Check sheet for the modelled part. Datum: model origin and axes. Units: mm. A direction names the side the tool comes from. Round coordinates to 2 decimals unless told otherwise and drop trailing zeros. Loops run counter-clockwise (first coordinate to the right, second up) from the corner with the lowest first, then second, coordinate; pieces in that order, holes last. Notation, with made-up numbers: (-24, 4) - (-2, 4) arc R12 ccw to (-2, 16) - close; hole circle Ø3 at (-14, 48.5). An arc over 180 degrees is marked (long way). Return JSON: item names as keys, results as strings.
from build123d import *

# Parameters (mm, degrees)
SKETCH_1_R          = 26
EXTRUDE_1_DEPTH     = 10
SKETCH_3_R          = 29
CUT_EXTRUDE_1_DEPTH = 6
SKETCH_4_W          = 40
SKETCH_4_H          = 12
EXTRUDE_2_DEPTH     = 12
SKETCH_5_W          = 40
SKETCH_5_H          = 12
EXTRUDE_3_DEPTH     = 2
SKETCH_6_W          = 40
SKETCH_6_H          = 12
EXTRUDE_4_DEPTH     = 3
CHAMFER_1_SIZE      = 14
SKETCH_7_R          = 1.7
CUT_EXTRUDE_2_DEPTH = 14
SKETCH_8_R          = 2.15
SKETCH_8_R_2        = 2.165
CUT_EXTRUDE_3_DEPTH = 6
SKETCH_9_W          = 40
SKETCH_9_H          = 12
CUT_EXTRUDE_4_DEPTH = 5
CHAMFER_2_SIZE      = 4
CHAMFER_3_SIZE      = 4
FILLET_5_R          = 10
FILLET_6_R          = 4
FILLET_7_R          = 3


with BuildPart() as part:
    # Sketch 1 → Extrude 1 (new body)
    with BuildSketch(Plane.XY):
        with BuildLine():
            Line((20, -27.158003748), (-20, -27.158003748))
            Line((-20, -27.158003748), (-20, 0.909194251))
            ThreePointArc((-20, 0.909194251), (0, 60.158003748), (20, 0.909194251))
            Line((20, 0.909194251), (20, -27.158003748))
        make_face()
        with Locations((0, 27.158003748)):
            Circle(SKETCH_1_R, mode=Mode.SUBTRACT)
    extrude(amount=EXTRUDE_1_DEPTH)

    # Sketch 3 → Cut-Extrude 1 (cut)
    with BuildSketch(Plane.XY.offset(10)):
        with Locations((0, 27.158003748)):
            Circle(SKETCH_3_R)
    extrude(amount=-CUT_EXTRUDE_1_DEPTH, mode=Mode.SUBTRACT)



with BuildPart() as body_2:
    # Sketch 4 → Extrude 2 (new body)
    with BuildSketch(Plane.XY.offset(10)):
        with Locations((0, -33.158003748)):
            Rectangle(SKETCH_4_W, SKETCH_4_H)
    extrude(amount=EXTRUDE_2_DEPTH)


with BuildPart() as part_1:
    add(part.part)

    add(body_2.part)  # Extrude 3 merges body 2
    # Sketch 5 → Extrude 3 (add)
    with BuildSketch(Plane(origin=(0, 0, 10), x_dir=(-1, 0, 0), z_dir=(0, 0, -1))):
        with Locations((0, -33.158003748)):
            Rectangle(SKETCH_5_W, SKETCH_5_H)
    extrude(amount=EXTRUDE_3_DEPTH)

    # Sketch 6 → Extrude 4 (add)
    with BuildSketch(Plane(origin=(0, -27.158003748, 0), x_dir=(1, 0, 0), z_dir=(0, 1, 0))):
        with Locations((0, -16)):
            Rectangle(SKETCH_6_W, SKETCH_6_H)
    extrude(amount=EXTRUDE_4_DEPTH)

    # Chamfer 1
    # the kernel refuses this chamfer: 14 mm, written as the material it adds along each edge
    with BuildSketch(Plane(origin=(-20, -24.158003748, 10), x_dir=(0, -0.027495876610586365, 0.9996219169112968), z_dir=(1, 0, 0))) as chamfer_1_piece_1_section:
        Polygon((CHAMFER_1_SIZE * 0.999621916911, -CHAMFER_1_SIZE * 0.0274958766106), (-CHAMFER_1_SIZE * 0.0274958766106, -CHAMFER_1_SIZE * 0.999621916911), (0, 0), align=None)
    chamfer_1_piece_1 = extrude(amount=40, mode=Mode.PRIVATE)
    chamfer_1_piece_1 = split(chamfer_1_piece_1, bisect_by=Plane(origin=(0, -19.403075602, 22), z_dir=(0, 0, -1)), keep=Keep.TOP, mode=Mode.PRIVATE)
    add(chamfer_1_piece_1)

    # Sketch 7 → Cut-Extrude 2 (cut)
    with BuildSketch(Plane(origin=(0, 0, 8), x_dir=(-1, 0, 0), z_dir=(0, 0, -1))):
        with Locations((-12, -33.833568363)):
            Circle(SKETCH_7_R)
        with Locations((12.012999622, -33.833568363)):
            Circle(SKETCH_7_R)
    extrude(amount=-CUT_EXTRUDE_2_DEPTH, mode=Mode.SUBTRACT)

    # Sketch 8 → Cut-Extrude 3 (cut)
    with BuildSketch(Plane.XY.offset(22)):
        with Locations((-12.012999622, -33.833568363)):
            Circle(SKETCH_8_R)
        with Locations((12, -33.833568363)):
            Circle(SKETCH_8_R_2)
    extrude(amount=-CUT_EXTRUDE_3_DEPTH, mode=Mode.SUBTRACT)

    # Sketch 9 → Cut-Extrude 4 (cut)
    with BuildSketch(Plane(origin=(0, 0, 8), x_dir=(-1, 0, 0), z_dir=(0, 0, -1))):
        with Locations((0, -33.158003748)):
            Rectangle(SKETCH_9_W, SKETCH_9_H)
    extrude(amount=-CUT_EXTRUDE_4_DEPTH, mode=Mode.SUBTRACT)

    # Chamfer 2
    # the kernel refuses this chamfer: 4 mm, written as the material it takes off along each edge
    with BuildSketch(Plane(origin=(30.286731952, -39.158003748, 22), x_dir=(0, 0.9996219169112968, 0.02749587661058651), z_dir=(-1, 0, 0))) as chamfer_2_piece_1:
        Polygon((CHAMFER_2_SIZE * 0.999621916911, CHAMFER_2_SIZE * 0.0274958766106), (-CHAMFER_2_SIZE * 0.0274958766106, CHAMFER_2_SIZE * 0.999621916911), (0, 0), align=None)
    extrude(amount=60.573463904, mode=Mode.SUBTRACT)

    # Chamfer 3
    chamfer_3_edges = [part_1.edges().sort_by_distance(p)[0] for p in [
        (0, -27.158003748, 0),
    ]]
    chamfer(chamfer_3_edges, length=CHAMFER_3_SIZE)

    # Fillet 5
    fillet_5_edges = [part_1.edges().sort_by_distance(p)[0] for p in [
        (-20, 0.909194251, 5),
        (20, 0.909194251, 5),
    ]]
    fillet(fillet_5_edges, radius=FILLET_5_R)

    # Fillet 6
    fillet_6_edges = [part_1.edges().sort_by_distance(p)[0] for p in [
        (0, 60.158003748, 0),
        (-20, -13.402921801, 0),
        (-20.786763819, 0.240126076, 0),
        (20.786763819, 0.240126076, 0),
        (20, -13.402921801, 0),
    ]]
    fillet(fillet_6_edges, radius=FILLET_6_R)

    # Fillet 7
    fillet_7_edges = [part_1.edges().sort_by_distance(p)[0] for p in [
        (0, -22.158003748, 22),
    ]]
    fillet(fillet_7_edges, radius=FILLET_7_R)


solid = part_1.part
Q1. Sectioned sample at B-B (y = -6). Enter the section's corners in (x, z).
Answer key:
{"outline": "(-20, 4) arc R4 ccw to (-16, 0) - (16, 0) arc R4 ccw to (20, 4) - (20, 10) - (-20, 10) - close"}
Q2. Sectioned sample at C-C (z = 8.75). Enter the section's corners in (x, y).
Answer key:
{"outline": "(-23.02, 3.52) arc R10 cw to (-20, -3.65) - (-20, -27.16) - (20, -27.16) - (20, -3.65) arc R10 cw to (23.02, 3.52) arc R33 ccw (long way) to start; hole circle Ø58 at (0, 27.16)"}
Q3. Tool access check on faces 4 (the face through (-10, -1, 10)), 5 (the face through (-11, 51, 4)), 6 (the face through (-18.797, -15.238, 1.141)). Record the directions out of +Z, -Z, +X, -X, +Y, -Y that give a thin tool (end or side, any length) a straight path to the whole face; none if there is none.
Answer key:
{"face 4": "+Z, +X, -X, +Y", "face 5": "+Z", "face 6": "-Z, -X, -Y"}
Q4. Scan lines: probe 1 along Z at (x, y) = (-9.5, 0); probe 2 along X at (y, z) = (1.5, 6.5); probe 3 along Y at (x, z) = (-4, 9.25). Record each from-to range of solid material in increasing order. Write a range as [from, to].
Answer key:
{"probe 1": "z = [0, 4]", "probe 2": "x = [-21.43, -13.52], [13.52, 21.43]", "probe 3": "y = [-27.16, -1.56], [55.88, 59.91]"}
Q5. Depth check by flat-ended pin: P1, Ø5, axis at y = 34, z = 3.5, coming from the -X side; P2, Ø10, axis at x = 9.5, z = 7.5, coming from the -Y side; P3, Ø2, axis at x = 6, y = -2, coming from the +Z side; P4, Ø12, axis at y = 28.5, z = 16.5, coming from the +X side. Enter the tip coordinate at first touch or a pass-through.
Answer key:
{"P1": "stops at x = -32.71", "P2": "stops at y = -27.16", "P3": "stops at z = 10", "P4": "passes through"}
Q6. Draft check along X on faces 1 (the face through (20, -22, 13)), 2 (the face through (-14, -34, 16)), 3 (the face through (0, -29, 22)). Enter one of: released by +X, released by -X, zero draft, split by the parting line, or undercut.
Answer key:
{"face 1": "released by +X", "face 2": "undercut", "face 3": "zero draft"}
Q7. Sectioned sample at A-A (x = 0). Enter the section's corners in (y, z).
Answer key:
{"outline": "(-39.16, 13) - (-27.16, 13) - (-27.16, 4) - (-23.16, 0) - (1.16, 0) - (1.16, 4) - (-1.84, 4) - (-1.84, 10) - (-10.16, 10) - (-21.28, 21.12) arc R3 ccw to (-23.4, 22) - (-35.16, 22) - (-39.16, 18) - close; (53.16, 0) - (56.16, 0) arc R4 ccw to (60.16, 4) - (60.16, 10) - (56.16, 10) - (56.16, 4) - (53.16, 4) - close"}
Q8. Sectioned sample at D-D (x = 12). State how many separate pieces and enclosed holes the cut face has, plus the area to 3 significant figures.
Answer key:
{"separate pieces": "3", "enclosed holes": "0", "area": "534 mm²"}
